from build123d import *

# Parameters (mm, degrees)
PAD_DEPTH     = 12.9
SKETCH001_R   = 6
PAD001_DEPTH  = 1.5
SKETCH002_R   = 2.9
SKETCH002_R_2 = 0.95
POCKET_DEPTH  = 10
FILLET_R      = 0.6
CHAMFER_SIZE  = 0.7
SKETCH003_R   = 0.2
PAD002_DEPTH  = 0.2


with BuildPart() as part:
    # Sketch → Pad (new body)
    with BuildSketch(Plane.XZ):
        with BuildLine():
            Line((4.4, -3.130495), (4.4, 3.130495))
            ThreePointArc((4.4, 3.130495), (-5.4, 0), (4.4, -3.130495))
        make_face()
    extrude(amount=-PAD_DEPTH)

    # Sketch001 (on Face3 of Pad) → Pad001 (join)
    with BuildSketch(Plane.XZ):
        Circle(SKETCH001_R)
    extrude(amount=PAD001_DEPTH)

    # Sketch002 (on Face3 of Pad001) → Pocket (cut)
    with BuildSketch(Plane.XZ.offset(1.5)):
        Circle(SKETCH002_R)
        Circle(SKETCH002_R_2, mode=Mode.SUBTRACT)
    extrude(amount=-POCKET_DEPTH, mode=Mode.SUBTRACT)

    # Fillet
    fillet_edges = [part.edges().sort_by_distance(p)[0] for p in [
        (-0.95, -1.5, 0),
    ]]
    fillet(fillet_edges, radius=FILLET_R)

    # Chamfer
    chamfer_edges = [part.edges().sort_by_distance(p)[0] for p in [
        (-6, -1.5, 0),
    ]]
    chamfer(chamfer_edges, length=CHAMFER_SIZE)

    # Sketch003 (on Face8 of Chamfer) → Pad002 (join)
    with BuildSketch(Plane(origin=(4.4, 0, 0), x_dir=(0, 0, 1), z_dir=(1, 0, 0))):
        with BuildLine():
            Line((0.8, -12.9), (-0.8, -12.9))
            Line((-0.8, -12.9), (-0.8, -15.9))
            ThreePointArc((-0.8, -15.9), (0, -16.7), (0.8, -15.9))
            Line((0.8, -15.9), (0.8, -12.9))
        make_face()
        with Locations((0, -15.9)):
            Circle(SKETCH003_R, mode=Mode.SUBTRACT)
    pad002 = extrude(amount=-PAD002_DEPTH)

    # Mirrored: Pad002 across YZ
    add(pad002.mirror(Plane.YZ))


solid = part.part
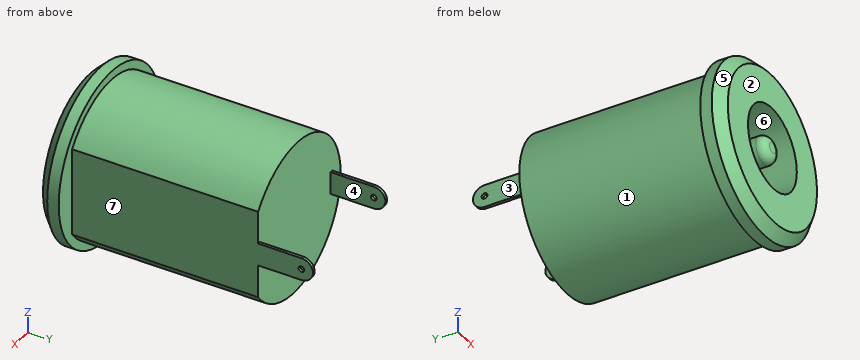
Here's how the part is built. I have some questions about the finished solid (model axes, mm). Face numbers are marked on the shaded views. A direction names the side the tool comes from. Coordinates: 2 decimals unless noted, no trailing zeros. Write each loop counter-clockwise with the first axis right and the second up, starting at its lowest first coordinate (ties: lowest second). Pieces come first, ordered by that corner, then holes.
1) Which directions (+Z, -Z, +X, -X, +Y, -Y) give clear straight access to the entire face, cutting with the end or side of a thin tool? Please do the marked faces 1, 2 and 3.
Filled in:
face 1: +Y
face 2: +Z, -Z, +X, -X, -Y
face 3: +Z, -Z, -X, +Y
2) If we section it at B-B (z = 0): Count the separate pieces of the cut face and the enclosed holes in it, plus the area to 3 significant figures.
Filled in:
separate pieces: 3
enclosed holes: 0
area: 106 mm2
3) If I drill on line 1 (Z direction, x = 0, y = 6.75); line 2 (Z direction, x = 4.3, y = 15.9); line 3 (Y direction, x = 4.3, z = 0), over which ranges is the centre line in solid material (lowest first)?
Filled in:
line 1: z = -5.4 to -2.9, -0.95 to 0.95, 2.9 to 5.4
line 2: z = -0.8 to -0.2, 0.2 to 0.8
line 3: y = -1.5 to 15.7, 16.1 to 16.7
4) Thinking about a two-plate mould opening in X: for the marked faces 4, 5, 6 and 7, which applies, +X half, -X half, draft (parallel to the pull), parting line (faces both ways), or undercut?
Filled in:
face 4: undercut
face 5: parting line
face 6: undercut
face 7: +X half
5) If we section it at A-A (y = 15): List the corners of the cut face in (x, z) for me.
Filled in:
outline: (-4.4, -0.8) - (-4.2, -0.8) - (-4.2, 0.8) - (-4.4, 0.8) - close; (4.2, -0.8) - (4.4, -0.8) - (4.4, 0.8) - (4.2, 0.8) - close
6) I'm going to push flat-ended pins straight in: pin 1 (0.8 mm diameter, centred on y = 14, z = 0, fed in from -X); pin 2 (1.5 mm diameter, centred on x = 0, y = 7.5, fed in from +Z); pin 3 (3 mm diameter, centred on x = 1, z = 0.5, fed in from -Y); pin 4 (1.5 mm diameter, centred on x = 3.5, y = 3.5, fed in from -Z). Where does each tip first touch, or does it pass through?
Filled in:
pin 1: stops at x = -4.4
pin 2: stops at z = 5.4
pin 3: stops at y = -1.5
pin 4: stops at z = -4.65
7) If we section it at C-C (y = 3.5): List the corners of the cut face in (x, z) for me, plus the area to 3 significant figures.
Filled in:
outline: circle Ø1.9 at (0, 0); (4.4, -3.13) - (4.4, 3.13) arc R5.4 ccw (long way) to start; hole circle Ø5.8 at (0, 0)
area: 63.8 mm2
